```python
from build123d import *

# Parameters (mm, degrees)
SKETCH1_W             = 345
SKETCH1_H             = 125
SKETCH1_R             = 8.5
BOSS_EXTRUDE1_DEPTH   = 10
SKETCH1_3_R           = 8.5
CUT_EXTRUDE1_DEPTH    = 184.74574825
CRVPATTERN1_OUTLINE_R = 8.5
CRVPATTERN1_DEPTH     = 10


# Read off the part's stored shape, not the designer's step: CrvPattern1
with BuildPart() as part:
    # Sketch1 → Boss-Extrude1 (new body)
    # profile 1 of 2: a face of its own
    with BuildSketch(Plane(origin=(0, 0, 0), x_dir=(1, 0, 0), z_dir=(0, 1, 0))):
        Rectangle(SKETCH1_W, SKETCH1_H)
        with Locations((-143, 37.5)):
            Circle(SKETCH1_R, mode=Mode.SUBTRACT)
    # profile 2 of 2: a face of its own
    with BuildSketch(Plane(origin=(0, 0, 0), x_dir=(1, 0, 0), z_dir=(0, 1, 0))):
        with Locations((-143, 37.5)):
            Circle(SKETCH1_R)
    extrude(amount=BOSS_EXTRUDE1_DEPTH)

    # Sketch1<3> → Cut-Extrude1 (cut, through all)
    with BuildSketch(Plane(origin=(0, 0, 0), x_dir=(1, 0, 0), z_dir=(0, 1, 0))):
        with Locations(Location((-143, 37.5, 0), (0, 0, 270))):
            Circle(SKETCH1_3_R)
    extrude(amount=CUT_EXTRUDE1_DEPTH, mode=Mode.SUBTRACT)

    # CrvPattern1 outline → CrvPattern1 (cut)
    with BuildSketch(Plane(origin=(0, 0, 0), x_dir=(1, 0, 0), z_dir=(0, 1, 0))):
        with Locations((-143, 12.5)):
            Circle(CRVPATTERN1_OUTLINE_R)
        with Locations((143, 12.5)):
            Circle(CRVPATTERN1_OUTLINE_R)
        with Locations((143, 37.5)):
            Circle(CRVPATTERN1_OUTLINE_R)
        with Locations((114.4, -37.5)):
            Circle(CRVPATTERN1_OUTLINE_R)
        with Locations((114.4, -12.5)):
            Circle(CRVPATTERN1_OUTLINE_R)
        with Locations((114.4, 12.5)):
            Circle(CRVPATTERN1_OUTLINE_R)
        with Locations((114.4, 37.5)):
            Circle(CRVPATTERN1_OUTLINE_R)
        with Locations((85.8, -37.5)):
            Circle(CRVPATTERN1_OUTLINE_R)
        with Locations((85.8, -12.5)):
            Circle(CRVPATTERN1_OUTLINE_R)
        with Locations((143, -12.5)):
            Circle(CRVPATTERN1_OUTLINE_R)
        with Locations((143, -37.5)):
            Circle(CRVPATTERN1_OUTLINE_R)
        with Locations((-85.8, -12.5)):
            Circle(CRVPATTERN1_OUTLINE_R)
        with Locations((-85.8, -37.5)):
            Circle(CRVPATTERN1_OUTLINE_R)
        with Locations((-57.2, 37.5)):
            Circle(CRVPATTERN1_OUTLINE_R)
        with Locations((-57.2, 12.5)):
            Circle(CRVPATTERN1_OUTLINE_R)
        with Locations((-57.2, -12.5)):
            Circle(CRVPATTERN1_OUTLINE_R)
        with Locations((-57.2, -37.5)):
            Circle(CRVPATTERN1_OUTLINE_R)
        with Locations((-28.6, 37.5)):
            Circle(CRVPATTERN1_OUTLINE_R)
        with Locations((-28.6, 12.5)):
            Circle(CRVPATTERN1_OUTLINE_R)
        with Locations((-143, -12.5)):
            Circle(CRVPATTERN1_OUTLINE_R)
        with Locations((-143, -37.5)):
            Circle(CRVPATTERN1_OUTLINE_R)
        with Locations((-114.4, 37.5)):
            Circle(CRVPATTERN1_OUTLINE_R)
        with Locations((-114.4, 12.5)):
            Circle(CRVPATTERN1_OUTLINE_R)
        with Locations((-114.4, -12.5)):
            Circle(CRVPATTERN1_OUTLINE_R)
        with Locations((-114.4, -37.5)):
            Circle(CRVPATTERN1_OUTLINE_R)
        with Locations((-85.8, 37.5)):
            Circle(CRVPATTERN1_OUTLINE_R)
        with Locations((-85.8, 12.5)):
            Circle(CRVPATTERN1_OUTLINE_R)
        with Locations((28.6, -12.5)):
            Circle(CRVPATTERN1_OUTLINE_R)
        with Locations((28.6, -37.5)):
            Circle(CRVPATTERN1_OUTLINE_R)
        with Locations((57.2, 37.5)):
            Circle(CRVPATTERN1_OUTLINE_R)
        with Locations((57.2, 12.5)):
            Circle(CRVPATTERN1_OUTLINE_R)
        with Locations((57.2, -12.5)):
            Circle(CRVPATTERN1_OUTLINE_R)
        with Locations((57.2, -37.5)):
            Circle(CRVPATTERN1_OUTLINE_R)
        with Locations((85.8, 37.5)):
            Circle(CRVPATTERN1_OUTLINE_R)
        with Locations((85.8, 12.5)):
            Circle(CRVPATTERN1_OUTLINE_R)
        with Locations((-28.6, -12.5)):
            Circle(CRVPATTERN1_OUTLINE_R)
        with Locations((-28.6, -37.5)):
            Circle(CRVPATTERN1_OUTLINE_R)
        with Locations((0, 37.5)):
            Circle(CRVPATTERN1_OUTLINE_R)
        with Locations((0, 12.5)):
            Circle(CRVPATTERN1_OUTLINE_R)
        with Locations((0, -12.5)):
            Circle(CRVPATTERN1_OUTLINE_R)
        with Locations((0, -37.5)):
            Circle(CRVPATTERN1_OUTLINE_R)
        with Locations((28.6, 37.5)):
            Circle(CRVPATTERN1_OUTLINE_R)
        with Locations((28.6, 12.5)):
            Circle(CRVPATTERN1_OUTLINE_R)
    extrude(amount=CRVPATTERN1_DEPTH, mode=Mode.SUBTRACT)


solid = part.part
```
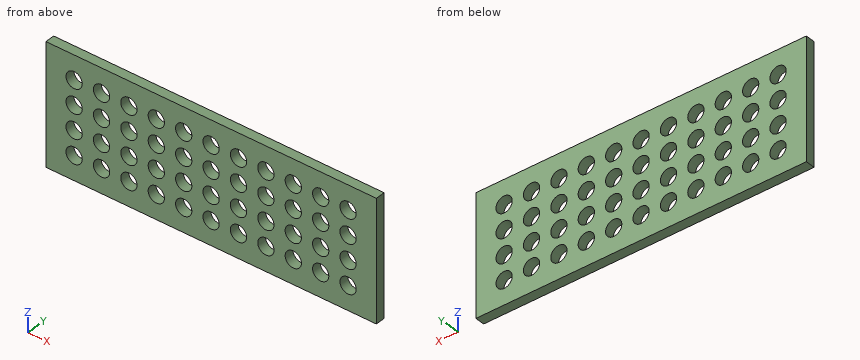
Here's how the part is built. I have some questions about the finished solid (model axes, mm). Coordinates: 2 decimals unless noted, no trailing zeros. Loops run counter-clockwise (first coordinate to the right, second up) from the corner with the lowest first, then second, coordinate; pieces in that order, holes last. Notation, with made-up numbers: (32.25, -34) -> (79.25, -34) arc R28 cw to (79.25, -6) -> close; hole circle Ø2 at (59, 42.25). An arc over 180 degrees is marked (long way). Return JSON: item names as keys, results as strings.
1) If we section it at B-B, the plane z = -33.5: Count the separate pieces of the cut face and the enclosed holes in it, then the cut area to 3 significant figures.
Results below:
{"separate pieces": "12", "enclosed holes": "0", "area": "1,800 mm²"}
2) If we section it at D-D, the plane x = 142: Write out the boundary of the cut face in (y, z).
Results below:
{"outline": "(0, -62.5) -> (10, -62.5) -> (10, -45.94) -> (0, -45.94) -> close; (0, -29.06) -> (10, -29.06) -> (10, -20.94) -> (0, -20.94) -> close; (0, -4.06) -> (10, -4.06) -> (10, 4.06) -> (0, 4.06) -> close; (0, 20.94) -> (10, 20.94) -> (10, 29.06) -> (0, 29.06) -> close; (0, 45.94) -> (10, 45.94) -> (10, 62.5) -> (0, 62.5) -> close"}
3) If we section it at A-A, the plane x = -57.2: Write out the boundary of the cut face in (y, z), then the cut area to 3 significant figures.
Results below:
{"outline": "(0, -62.5) -> (10, -62.5) -> (10, -46) -> (0, -46) -> close; (0, -29) -> (10, -29) -> (10, -21) -> (0, -21) -> close; (0, -4) -> (10, -4) -> (10, 4) -> (0, 4) -> close; (0, 21) -> (10, 21) -> (10, 29) -> (0, 29) -> close; (0, 46) -> (10, 46) -> (10, 62.5) -> (0, 62.5) -> close", "area": "570 mm²"}
4) I need wall thicknesses on line 1 (Z direction, x = -143, y = 2.5); line 2 (Z direction, x = -148, y = 4.5). Which ranges of each line are inside material? Lowest first, please. Write a range as from..to.
Results below:
{"line 1": "-62.5..-46, -29..-21, -4..4, 21..29, 46..62.5", "line 2": "-62.5..-44.37, -30.63..-19.37, -5.63..5.63, 19.37..30.63, 44.37..62.5"}
5) Will this pin go through, and if not, where does the flat tip stop? pin 1 (13.5 mm diameter, centred on x = 57.2, z = -37.5, fed in from -Y).
Results below:
{"pin 1": "through"}
